Here's how the part is built. I have some questions about the finished solid (model axes, mm). Face numbers are marked on the shaded views. A direction names the side the tool comes from. Round coordinates to 2 decimals unless told otherwise and drop trailing zeros. Write each loop counter-clockwise with the first axis right and the second up, starting at its lowest first coordinate (ties: lowest second). Pieces come first, ordered by that corner, then holes. Notation, with made-up numbers: M 31,-32.75 L 58,-32.75 A11 ccw 58,-15.75 Z; hole C -22,28 d7. An arc over 180 degrees is marked long. Use a Markdown table: item, result. Add a question column.
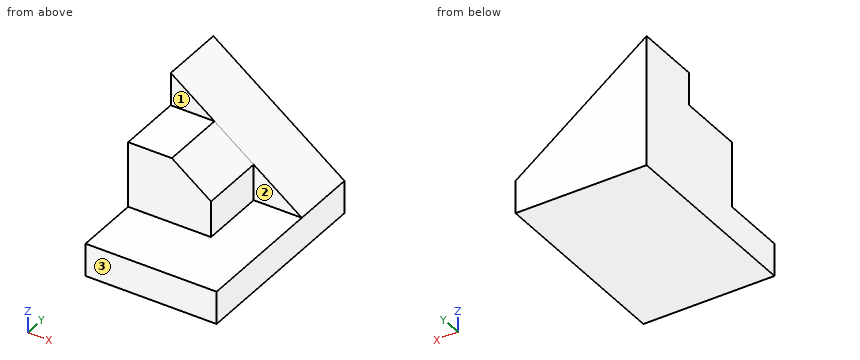
```python
from build123d import *

# Parameters (mm, degrees)
F0_W     = 25.4
F0_H     = 6.35
F1_DEPTH = 38.1
F3_DEPTH = 12.7
F5_DEPTH = 12.7


with BuildPart() as f1:
    # F0 (on Front) → F1 (new body)
    with BuildSketch(Plane.XZ):
        with Locations((12.7, 3.175)):
            Rectangle(F0_W, F0_H)
    extrude(amount=-F1_DEPTH)

    # F2 (on face) → F3 (join)
    with BuildSketch(Plane(origin=(0, 38.1, 0), x_dir=(-1, 0, 0), z_dir=(0, 1, 0))):
        Polygon((-25.4, 6.35), (0, 6.35), (0, 25.4), align=None)
    extrude(amount=-F3_DEPTH)

    # F4 (on face) → F5 (join)
    with BuildSketch(Plane.XZ.offset(-25.4)):
        Polygon((0, 19.05), (0, 6.35), (16.062235, 6.35), (16.062235, 13.353323), (8.466667, 19.05), align=None)
    extrude(amount=F5_DEPTH)


solid = f1.part
```
Item 1: Imagine slicing it at A-A on z = 7.25. List the corners of the cut face in (x, y) for me, plus the area to 3 significant figures.
Item 2: For pin 1 Ø3 at (x, z) = (6, 22.5) entering from -Y; pin 2 Ø3.5 at (y, z) = (20, 9.5) entering from +X; pin 3 Ø6 at (x, z) = (12, 14.5) entering from -Y, each with a flat end and sliding along its axis, tell me the tip position at first contact or that it passes through.
Item 3: Imagine slicing it at B-B on y = 21. List the corners of the cut face in (x, z) for me, plus the area to 3 significant figures.
Item 4: Imagine slicing it at C-C on x = 5.5. List the corners of the cut face in (y, z) for me (3 decimals).
Item 5: Imagine slicing it at D-D on x = 20.75. List the corners of the cut face in (y, z) for me.
Item 6: I need wall thicknesses on probe 1 along Z at (x, y) = (20.75, 18.5); probe 2 along Y at (x, z) = (3, 17.5); probe 3 along X at (y, z) = (17, 7.75). Which ranges of each line are inside material? Lowest first, please. Write a range as from..to.
Item 7: On a 3-axis mill with a long thin cutter (end or side, diameter ignored), from which of +Z, -Z, +X, -X, +Y, -Y can I reach the whole of each face in a straight line? I mean the marked faces 1, 2 and 3. Say none if no direction works.
The answers:
| question | item | result |
|---|---|---|
| 1 | outline | M 0,12.7 L 16.06,12.7 L 16.06,25.4 L 24.2,25.4 L 24.2,38.1 L 0,38.1 Z |
| 1 | area | 511 mm² |
| 2 | pin 1 | y = 25.4 |
| 2 | pin 2 | x = 16.06 |
| 2 | pin 3 | y = 12.7 |
| 3 | outline | M 0,0 L 25.4,0 L 25.4,6.35 L 16.06,6.35 L 16.06,13.35 L 8.47,19.05 L 0,19.05 Z |
| 3 | area | 344 mm² |
| 4 | outline | M 0,0 L 38.1,0 L 38.1,21.275 L 25.4,21.275 L 25.4,19.05 L 12.7,19.05 L 12.7,6.35 L 0,6.35 Z |
| 5 | outline | M 0,0 L 38.1,0 L 38.1,9.84 L 25.4,9.84 L 25.4,6.35 L 0,6.35 Z |
| 6 | probe 1 | 0..6.35 |
| 6 | probe 2 | 12.7..38.1 |
| 6 | probe 3 | 0..16.06 |
| 7 | face 1 | +Z, +X, -X, -Y |
| 7 | face 2 | +Z, +X, -Y |
| 7 | face 3 | +Z, -Z, +X, -X, -Y |
